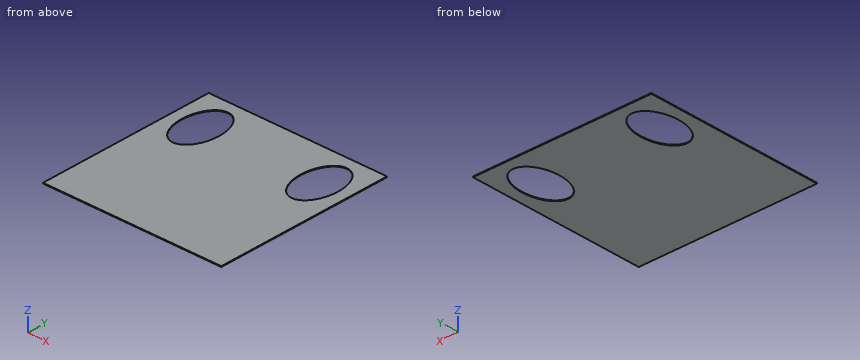
from build123d import *

# Parameters (mm, degrees)
SKETCH1_W           = 609.6
SKETCH1_H           = 609.6
BOSS_EXTRUDE1_DEPTH = 2.54
SKETCH2_RX          = 101.6
SKETCH2_RY          = 63.5
CUT_EXTRUDE1_DEPTH  = 3.54


with BuildPart() as part:
    # Sketch1 → Boss-Extrude1 (new body)
    with BuildSketch(Plane.XY):
        with Locations((120.912396694, -5.667768595)):
            Rectangle(SKETCH1_W, SKETCH1_H)
    extrude(amount=BOSS_EXTRUDE1_DEPTH)

    # Sketch2 → Cut-Extrude1 (cut, through all)
    with BuildSketch(Plane.XY.offset(2.54)):
        with Locations(Location((-82.287603306, 159.432231405), (0, 0, -90))):
            Ellipse(SKETCH2_RX, SKETCH2_RY)
        with Locations(Location((324.112396694, 159.432231405), (0, 0, -90))):
            Ellipse(SKETCH2_RX, SKETCH2_RY)
    extrude(amount=-CUT_EXTRUDE1_DEPTH, mode=Mode.SUBTRACT)


solid = part.part
Part model, mm, in its own coordinate system. Round coordinates to 2 decimals unless told otherwise and drop trailing zeros. Return JSON: item names as keys, results as strings. Group by question number.
(1) Pin check, flat tip, straight feed: pin 1 Ø12 at (x, y) = (190, -67.5) entering from -Z. Stop position of the tip, or through.
(2) Drill centre lines: probe 1 along X at (y, z) = (241.5, 1.35); probe 2 along X at (y, z) = (104, 1.35); probe 3 along Y at (x, z) = (276, 0.85). Where is each one in solid material? Low to high.
(3) Saw through at A-A on y = 124. Count the separate pieces of the cut face and the enclosed holes in it, then the cut area to 3 significant figures.
Returned:
{
 "1": {"pin 1": "z = 0"},
 "2": {"probe 1": "-183.89 to -119.72, -44.85 to 286.68, 361.55 to 425.71", "probe 2": "-183.89 to -135.5, -29.07 to 270.9, 377.33 to 425.71", "probe 3": "-310.47 to 93.12, 225.74 to 299.13"},
 "3": {"separate pieces": "3", "enclosed holes": "0", "area": "944 mm²"}
}
